Part model, mm, in its own coordinate system. Coordinates: 2 decimals unless noted, no trailing zeros. Order: outer loops, then holes, each group sorted by start corner. A loop starts at its lowest first (then second) coordinate and runs counter-clockwise, first axis right, second up.
1) Cut at B-B (x = 28). List the corners of the cut face in (y, z), and give its area (3 significant figures).
2) Cut at A-A (y = 6.5). List the corners of the cut face in (x, z).
3) Pin check, flat tips, straight feed: pin 1 Ø1 at (x, y) = (19, 80) entering from -Z; pin 2 Ø0.9 at (x, z) = (-2, 2) entering from -Y; pin 3 Ø1.5 at (x, z) = (20.5, 1) entering from +Y; pin 4 Ø1.5 at (y, z) = (-2, 1) entering from -X. Stop position of each tip, or through.
4) Wall check: L1, parallel to Y at x = 23, z = 2.65; L2, parallel to Y at x = 56.5, z = 2.25. Give the ranges that are in metal, low to high.
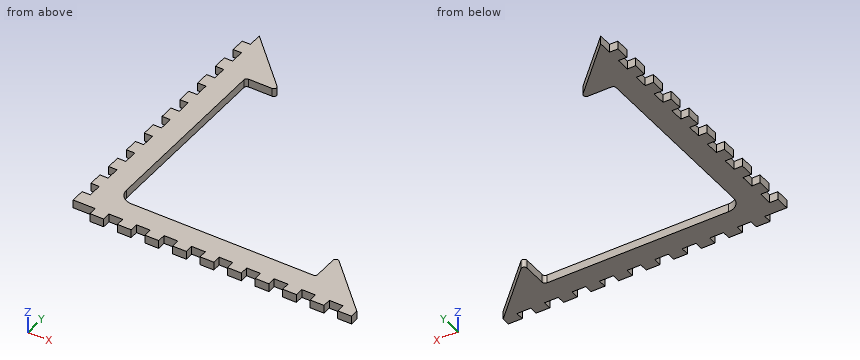
```python
from build123d import *

# Parameters (mm, degrees)
F1_DEPTH = 3
F3_W     = 3
F3_H     = 5
F2_W     = 5
F2_H     = 3
F4_DEPTH = 3
F5_R     = 1
F6_R     = 5


with BuildPart() as f1:
    # F0 (on Top) → F1 (new body)
    with BuildSketch(Plane.XY):
        Polygon((20, 80), (0, 100), (0, 0), (100, 0), (80, 20), (80, 8), (8, 8), (8, 80), align=None)
    extrude(amount=F1_DEPTH)

    # F3 (on face) + F2 (on face) → F4 (join)
    with BuildSketch(Plane.XY.offset(3)):
        with Locations((-1.5, 42.5)):
            Rectangle(F3_W, F3_H)
        with Locations((-1.5, 32.5)):
            Rectangle(F3_W, F3_H)
        with Locations((-1.5, 22.5)):
            Rectangle(F3_W, F3_H)
        with Locations((-1.5, 12.5)):
            Rectangle(F3_W, F3_H)
        with Locations((-1.5, 2.5)):
            Rectangle(F3_W, F3_H)
        with Locations((-1.5, 52.5)):
            Rectangle(F3_W, F3_H)
        with Locations((-1.5, 72.5)):
            Rectangle(F3_W, F3_H)
        with Locations((-1.5, 82.5)):
            Rectangle(F3_W, F3_H)
        with Locations((-1.5, 92.5)):
            Rectangle(F3_W, F3_H)
        with Locations((-1.5, 62.5)):
            Rectangle(F3_W, F3_H)
    with BuildSketch(Plane.XY.offset(3)):
        with Locations((7.5, -1.5)):
            Rectangle(F2_W, F2_H)
        with Locations((17.5, -1.5)):
            Rectangle(F2_W, F2_H)
        with Locations((27.5, -1.5)):
            Rectangle(F2_W, F2_H)
        with Locations((37.5, -1.5)):
            Rectangle(F2_W, F2_H)
        with Locations((47.5, -1.5)):
            Rectangle(F2_W, F2_H)
        with Locations((57.5, -1.5)):
            Rectangle(F2_W, F2_H)
        with Locations((67.5, -1.5)):
            Rectangle(F2_W, F2_H)
        with Locations((77.5, -1.5)):
            Rectangle(F2_W, F2_H)
        with Locations((87.5, -1.5)):
            Rectangle(F2_W, F2_H)
        with Locations((97.5, -1.5)):
            Rectangle(F2_W, F2_H)
    extrude(amount=-F4_DEPTH)

    # F5
    f5_edges = [f1.edges().sort_by_distance(p)[0] for p in [
        (80, 20, 1.5),
        (8, 80, 1.5),
        (20, 80, 1.5),
        (80, 8, 1.5),
    ]]
    fillet(f5_edges, radius=F5_R)

    # F6
    f6_edges = [f1.edges().sort_by_distance(p)[0] for p in [
        (8, 8, 1.5),
    ]]
    fillet(f6_edges, radius=F6_R)


solid = f1.part
```
Geometry check:
1. outline: (-3, 0) - (8, 0) - (8, 3) - (-3, 3) - close
1. area: 33.0 mm2
2. outline: (0, 0) - (93.5, 0) - (93.5, 3) - (0, 3) - close
3. pin 1: passes through
3. pin 2: stops at y = 0
3. pin 3: stops at y = 8
3. pin 4: stops at x = 5
4. L1: y = 0 to 8
4. L2: y = -3 to 8
